Part model, mm, in its own coordinate system. Face numbers are marked on the shaded views. A direction names the side the tool comes from. Coordinates: 2 decimals unless noted, no trailing zeros. Loops run counter-clockwise (first coordinate to the right, second up) from the corner with the lowest first, then second, coordinate; pieces in that order, holes last. Notation, with made-up numbers: M 77,25.25 L 111,25.25 A18 ccw 111,32.25 Z; hole C 15.5,30.5 d9. An arc over 180 degrees is marked long. Answer as CSV lines item,"result". Start each with the question number.
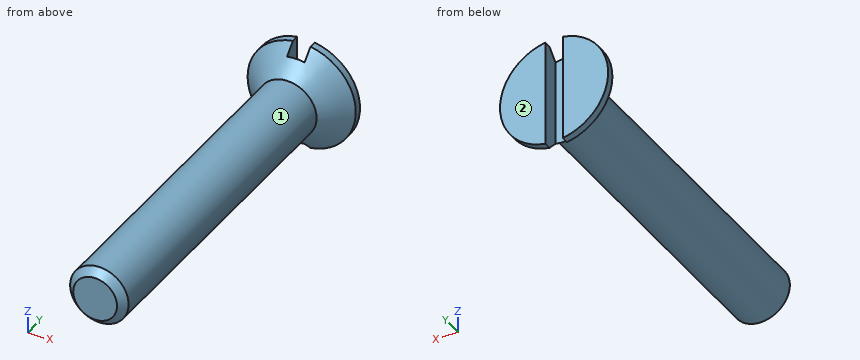
from build123d import *

# Parameters (mm, degrees)
CUT_EXTRUDE_1_DEPTH      = 26.54173056
CUT_EXTRUDE_1_DEPTH_BACK = 26.54173056
SKETCH_2_W               = 1.2
SKETCH_2_H               = 1.2


with BuildPart() as part:
    # Эскиз1 → Повернуть1 (revolve)
    with BuildSketch(Plane.XY):
        Polygon((0, 0), (-1.5, 0), (-2, 0.5), (-2, 22.8), (-3.7, 24.5), (-3.7, 25), (0, 25), align=None)
    revolve(axis=Axis((0, 25, 0), (0, -1, 0)))

    # Эскиз2 → Вырез-Вытянуть1 (cut, two sides: drawn at the far end of the back side and taken through both)
    with BuildSketch(Plane.XY.offset(-CUT_EXTRUDE_1_DEPTH_BACK)):
        with Locations((0, 24.4)):
            Rectangle(SKETCH_2_W, SKETCH_2_H)
    extrude(amount=CUT_EXTRUDE_1_DEPTH + CUT_EXTRUDE_1_DEPTH_BACK, mode=Mode.SUBTRACT)


solid = part.part
Q1. Wall check: L1, parallel to Z at x = 0, y = 8; L2, parallel to Y at x = -0.5, z = -0.5; L3, parallel to X at y = 21.75, z = -1. Give the ranges that are in metal, low to high.
Q2. Slice it at B-B, the plane x = 0. Write the cut outline in (y, z), and give its area (4 significant figures).
Q3. Slice it at C-C, the plane y = 12.75. Write the cut outline in (x, z), and give its area (3 significant figures).
Q4. Slice it at A-A, the plane z = 0. Write the cut outline in (x, y).
Q5. Tool access for the marked faces 1 and 2: list every direction of +Z, -Z, +X, -X, +Y, -Y with a clear straight run to the whole face (end or side of a thin tool).
Q6. Flat gauge pins, fed straight in: P1, Ø3, axis at x = -1.5, y = 6, coming from the -Z side; P2, Ø1.5, axis at y = 13.5, z = 0.5, coming from the -X side; P3, Ø0.6, axis at x = 0, z = -1, coming from the +Y side. Where does each tip first touch, or does it go through?
Solved:
1,L1,"z = -2 to 2"
1,L2,"y = 0 to 23.8"
1,L3,"x = -1.73 to 1.73"
2,outline,"M 0,-1.5 L 0.5,-2 L 22.8,-2 L 23.8,-3 L 23.8,3 L 22.8,2 L 0.5,2 L 0,1.5 Z"
2,area,"95.95 mm2"
3,outline,"C 0,0 d4"
3,area,"12.6 mm2"
4,outline,"M -3.7,24.5 L -2,22.8 L -2,0.5 L -1.5,0 L 1.5,0 L 2,0.5 L 2,22.8 L 3.7,24.5 L 3.7,25 L 0.6,25 L 0.6,23.8 L -0.6,23.8 L -0.6,25 L -3.7,25 Z"
5,face 1,"-Y"
5,face 2,"+Z, -Z, +X, -X, +Y"
6,P1,"stops at z = -2"
6,P2,"stops at x = -2"
6,P3,"stops at y = 23.8"
